Source: CAD feature listing. Evaluate the final solid. Frame: model axes, mm. Face numbers are marked on the shaded views. Round coordinates to 2 decimals unless told otherwise and drop trailing zeros. Order: outer loops, then holes, each group sorted by start corner. A loop starts at its lowest first (then second) coordinate and runs counter-clockwise, first axis right, second up. Notation, with made-up numbers: (-27, -28.75) - (24, -28.75) arc R22 ccw to (24, -12.75) - close; hole circle Ø10 at (85.5, 65.25). An arc over 180 degrees is marked (long way). Put each result on its own line as item: value. Start each with the question number.
1) Section C-C on y = 22. Output: boundary loops of the cut face in (x, z).
2) Contact query for flat-ended pins moving along their axis: P1, Ø0.9, axis at y = 16, z = 2, coming from the +X side; P2, Ø0.9, axis at y = 18.5, z = 2, coming from the -X side; P3, Ø1.5, axis at x = 16, y = 226, coming from the -Z side. Output: stop coordinate, or through.
3) Section B-B on z = 1.3. Output: boundary loops of the cut face in (x, y), then the cut area to 3 significant figures.
4) Section A-A on x = 50.5. Output: boundary loops of the cut face in (y, z).
5) Mould query, pull axis Z, two halves, no side actions, for the marked faces 1 and 2. Classes: +Z half, -Z half, draft (parallel to the pull), parting line (faces both ways), or undercut.
6) Line query: probe 1 along Y at (x, z) = (5.5, 1.9); probe 2 along X at (y, z) = (12, 1.05). Output: solid intervals per line, ascending. Write a range as [from, to].
```python
from build123d import *

# Parameters (mm, degrees)
EXTRUDE_1_DEPTH     = 3
SKETCH_4_W          = 15
SKETCH_4_H          = 21
CUT_EXTRUDE_1_DEPTH = 3


with BuildPart() as part:
    # 草图1 → 凸台-拉伸1 (new body)
    with BuildSketch(Plane.XY):
        Polygon((0, 240), (0, 265), (60, 265), (60, 240), (60, 0), (0, 0), align=None)
    extrude(amount=EXTRUDE_1_DEPTH)

    # 草图4 → 切除-拉伸1 (cut)
    with BuildSketch(Plane(origin=(0, 0, 0), x_dir=(-1, 0, 0), z_dir=(0, 0, -1))):
        with Locations((-52.5, 17.5)):
            Rectangle(SKETCH_4_W, SKETCH_4_H)
        with Locations((-7.5, 17.5)):
            Rectangle(SKETCH_4_W, SKETCH_4_H)
        with Locations((-7.5, 198.5)):
            Rectangle(SKETCH_4_W, SKETCH_4_H)
        with Locations((-52.5, 198.5)):
            Rectangle(SKETCH_4_W, SKETCH_4_H)
    extrude(amount=-CUT_EXTRUDE_1_DEPTH, mode=Mode.SUBTRACT)


solid = part.part
```
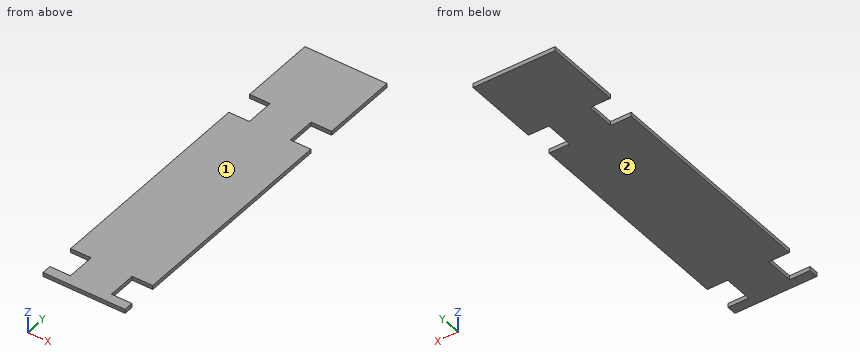
Answer sheet:
1. outline: (15, 0) - (45, 0) - (45, 3) - (15, 3) - close
2. P1: x = 45
2. P2: x = 15
2. P3: z = 0
3. outline: (0, 0) - (60, 0) - (60, 7) - (45, 7) - (45, 28) - (60, 28) - (60, 188) - (45, 188) - (45, 209) - (60, 209) - (60, 265) - (0, 265) - (0, 209) - (15, 209) - (15, 188) - (0, 188) - (0, 28) - (15, 28) - (15, 7) - (0, 7) - close
3. area: 14,600 mm^2
4. outline: (0, 0) - (7, 0) - (7, 3) - (0, 3) - close; (28, 0) - (188, 0) - (188, 3) - (28, 3) - close; (209, 0) - (265, 0) - (265, 3) - (209, 3) - close
5. face 1: +Z half
5. face 2: -Z half
6. probe 1: [0, 7], [28, 188], [209, 265]
6. probe 2: [15, 45]
